from build123d import *

# Parameters (mm, degrees)
BOSS_EXTRUDE1_DEPTH      = 175
FILLET1_R                = 10
CUT_EXTRUDE3_DEPTH       = 1129.731146152
CUT_EXTRUDE3_DEPTH_BACK  = 1129.731146152
SKETCH4_OUTSIDE_W        = 489.508
SKETCH4_OUTSIDE_H        = 264.508
FILLET4_R                = 10
BOSS_EXTRUDE2_REACH      = 261.692
BOSS_EXTRUDE2_END_RADIUS = 1097
BOSS_EXTRUDE3_REACH      = 261.692
BOSS_EXTRUDE3_END_RADIUS = 1097


with BuildPart() as part:
    # Sketch1 → Boss-Extrude1 (new body)
    with BuildSketch(Plane(origin=(0, 0, 0), x_dir=(1, 0, 0), z_dir=(0, 1, 0))):
        with BuildLine():
            Line((-200, -1068.442324134), (-200, -1078.614388927))
            ThreePointArc((-200, -1078.614388927), (0, -1097), (200, -1078.614388927))
            Line((200, -1078.614388927), (200, -1068.442324134))
            ThreePointArc((200, -1068.442324134), (0, -1087), (-200, -1068.442324134))
        make_face()
    extrude(amount=BOSS_EXTRUDE1_DEPTH)

    # Fillet1
    fillet1_edges = [part.edges().sort_by_distance(p)[0] for p in [
        (200, 175, 1073.52835653),
        (200, 0, 1073.52835653),
        (-200, 0, 1073.52835653),
    ]]
    fillet(fillet1_edges, radius=FILLET1_R)

    # Sketch4 outside → Cut-Extrude3 (cut, two sides: drawn at the far end of the back side and taken through both)
    with BuildSketch(Plane.XY.offset(-CUT_EXTRUDE3_DEPTH_BACK)):
        with Locations((0, 87.5)):
            Rectangle(SKETCH4_OUTSIDE_W, SKETCH4_OUTSIDE_H)
        Polygon((-190, 0), (50, 175), (-190, 175), align=None, mode=Mode.SUBTRACT)
    extrude(amount=CUT_EXTRUDE3_DEPTH + CUT_EXTRUDE3_DEPTH_BACK, mode=Mode.SUBTRACT)

    # Fillet4
    fillet4_edges = [part.edges().sort_by_distance(p)[0] for p in [
        (50, 175, 1090.854686691),
        (-190, 0, 1075.343303099),
        (-190, 175, 1075.343303099),
    ]]
    fillet(fillet4_edges, radius=FILLET4_R)

    # Boss-Extrude2: up to this cylinder (the profile starts outside it)
    boss_extrude2_end = Plane(origin=(0, 92.333894, 0), z_dir=(0, -1, 0)) * Cylinder(BOSS_EXTRUDE2_END_RADIUS, 2718.384, mode=Mode.PRIVATE)
    # Sketch5 → Boss-Extrude2 (add, up to the surface)
    with BuildSketch(Plane.XY.offset(1097), mode=Mode.PRIVATE) as boss_extrude2_sk1:
        with BuildLine():
            Line((-174.108278426, 11.587713648), (25.204468157, 156.919924698))
            ThreePointArc((25.204468157, 156.919924698), (28.820657842, 168.098325917), (19.312746583, 175))
            Line((19.312746583, 175), (-180, 175))
            ThreePointArc((-180, 175), (-187.071067812, 172.071067812), (-190, 165))
            Line((-190, 165), (-190, 19.66778895))
            ThreePointArc((-190, 19.66778895), (-184.53226126, 10.753833158), (-174.108278426, 11.587713648))
        make_face()
        Polygon((-180, 165), (-180, 19.66778895), (19.312746583, 165), align=None, mode=Mode.SUBTRACT)
    boss_extrude2_tool1 = extrude(boss_extrude2_sk1.sketch, amount=-BOSS_EXTRUDE2_REACH, mode=Mode.PRIVATE) - boss_extrude2_end
    add(boss_extrude2_tool1.solids().sort_by_distance((-187.253496, 92.333894, 1097))[0])
    add(boss_extrude2_tool1.solids().sort_by_distance((-187.253496, 92.333894, 1097))[1])

    # Boss-Extrude3: up to this cylinder (the profile starts outside it)
    boss_extrude3_end = Plane(origin=(0, 116.445193, 0), z_dir=(0, -1, 0)) * Cylinder(BOSS_EXTRUDE3_END_RADIUS, 2718.384, mode=Mode.PRIVATE)
    # Sketch6 → Boss-Extrude3 (add, up to the surface)
    with BuildSketch(Plane.XY.offset(1097), mode=Mode.PRIVATE) as boss_extrude3_sk1:
        Polygon((-11.374506835, 155), (-170, 155), (-170, 39.3355779), align=None)
    boss_extrude3_tool1 = extrude(boss_extrude3_sk1.sketch, amount=-BOSS_EXTRUDE3_REACH, mode=Mode.PRIVATE) - boss_extrude3_end
    add(boss_extrude3_tool1.solids().sort_by_distance((-117.124836, 116.445193, 1097))[0])


solid = part.part
Geometry: final body of the model. Coordinates: model frame, mm. A direction names the side the tool comes from. Round coordinates to 2 decimals unless told otherwise and drop trailing zeros. Loops run counter-clockwise (first coordinate to the right, second up) from the corner with the lowest first, then second, coordinate; pieces in that order, holes last.
Q1. Pull-direction query (X, two-part tool) for faces 1 (the flat face through (-101, 175, 1090)), 2 (the flat face through (-137.087, 50.959, 1092.905)), 3 (the flat face through (-180, 93, 1090)), 4 (the flat face through (-190, 93, 1084)); classes: released by +X, released by -X, zero draft, split by the parting line, or undercut.
Q2. Pin query (flat end, axial travel): P1, Ø3, axis at x = -51.5, z = 1090.5, coming from the -Y side; P2, Ø6, axis at x = -151.5, z = 1080.5, coming from the -Y side; P3, Ø12, axis at y = 78, z = 1091.5, coming from the +X side. Return the tip coordinate at first contact, or that it passes through.
Q3. Section B-B on y = 83. Return loops of the section in (x, z).
Q4. Section D-D on x = 14. Return loops of the section in (y, z).
Q5. Material intervals for L1, parallel to Y at x = -86.5, z = 1095; L2, parallel to Z at x = -119.5, y = 151; L3, parallel to X at y = 147.5, z = 1087.25, sorted ascending.
Q6. Access query for faces 5 (the flat face through (-109, 111, 1097)), 6 (the flat face through (-136, 165, 1092)). Directions: +Z, -Z, +X, -X, +Y, -Y. A direction counts if a zero-diameter tool reaches every point of the face in a straight line with its end or side. Return the directions, or none.
Q7. Section C-C on z = 1091.5. Return loops of the section in (x, y), plus the area to 3 significant figures.
Q8. Section A-A on x = -90. Return loops of the section in (y, z), plus the area to 3 significant figures.
Evaluation:
1. face 1: zero draft
1. face 2: undercut
1. face 3: undercut
1. face 4: released by -X
2. P1: stops at y = 99.9
2. P2: stops at y = 25.89
2. P3: stops at x = -74.8
3. outline: (-190, 1070.27) arc R1087 cw to (-76.17, 1084.33) - (-76.17, 1097) - (-93.14, 1097) - (-93.14, 1093.04) arc R1097 ccw to (-110.12, 1091.46) - (-110.12, 1097) - (-170, 1097) - (-170, 1083.75) arc R1097 ccw to (-180, 1082.13) - (-180, 1097) - (-190, 1097) - close
4. outline: (148.75, 1086.91) - (175, 1086.91) - (175, 1097) - (165, 1097) - (165, 1096.91) - (161.13, 1096.91) - (161.13, 1097) - (148.75, 1097) - close
5. L1: y = 75.47 to 87.84, 100.22 to 155, 165 to 175
5. L2: z = 1080.41 to 1097
5. L3: x = -190 to -180, -170 to 12.29
6. face 5: +Z, +X, -X, +Y, -Y
6. face 6: +Z
7. outline: (-190, 19.67) arc R10 ccw to (-174.11, 11.59) - (25.2, 156.92) arc R10 ccw to (19.31, 175) - (-180, 175) arc R10 ccw to (-190, 165) - close; hole (-180, 19.67) - (-109.71, 70.92) - (-109.71, 83.3) - (-170, 39.34) - (-170, 155) - (-109.71, 155) - (-109.71, 165) - (-180, 165) - close
7. area: 17,900 mm2
8. outline: (72.92, 1083.27) - (175, 1083.27) - (175, 1097) - (165, 1097) - (165, 1093.3) - (155, 1093.3) - (155, 1097) - (97.67, 1097) - (97.67, 1093.3) - (85.29, 1093.3) - (85.29, 1097) - (72.92, 1097) - close
8. area: 1,320 mm2
